```python
from build123d import *

# Parameters (mm, degrees)
SKETCH1_R           = 1.5
SKETCH1_W           = 16
SKETCH1_H           = 16
BOSS_EXTRUDE1_DEPTH = 4
BOSS_EXTRUDE2_START = 2
BOSS_EXTRUDE2_DEPTH = 2


with BuildPart() as part:
    # Sketch1 → Boss-Extrude1 (new body)
    with BuildSketch(Plane(origin=(0, 0, 0), x_dir=(1, 0, 0), z_dir=(0, 1, 0))):
        with BuildLine():
            Line((-2, 18), (18, 18))
            Line((18, 18), (18, -2))
            Line((18, -2), (-2, -2))
            Line((-2, -2), (-2, 4.5))
            Line((-2, 4.5), (-4, 4.5))
            ThreePointArc((-4, 4.5), (-7.5, 8), (-4, 11.5))
            Line((-4, 11.5), (-2, 11.5))
            Line((-2, 11.5), (-2, 18))
        make_face()
        with Locations(Location((-4, 8, 0), (0, 0, 270))):
            Circle(SKETCH1_R, mode=Mode.SUBTRACT)
        with Locations((8, 8)):
            Rectangle(SKETCH1_W, SKETCH1_H, mode=Mode.SUBTRACT)
    extrude(amount=BOSS_EXTRUDE1_DEPTH)

    # Sketch2 → Boss-Extrude2 (add)
    with BuildSketch(Plane.XZ.offset(BOSS_EXTRUDE2_START)):
        with BuildLine():
            Line((18, 2), (18, -18))
            Line((18, -18), (-2, -18))
            Line((-2, -18), (-2, -11.5))
            Line((-2, -11.5), (-4, -11.5))
            ThreePointArc((-4, -11.5), (-7.5, -8), (-4, -4.5))
            Line((-4, -4.5), (-2, -4.5))
            Line((-2, -4.5), (-2, 2))
            Line((-2, 2), (18, 2))
        make_face()
    extrude(amount=-BOSS_EXTRUDE2_DEPTH)


solid = part.part
```
The listing builds one solid part. Answer for the finished solid, in the listing's coordinates (mm). A direction names the side the tool comes from. Give positions to 0.01 mm unless a question says otherwise; leave off trailing zeros. Order: outer loops, then holes, each group sorted by start corner. A loop starts at its lowest first (then second) coordinate and runs counter-clockwise, first axis right, second up. Notation, with made-up numbers: (4.25, 63.5) - (63.25, 63.5) arc R13 ccw to (63.25, 75.5) - close; hole circle Ø4 at (80, 56.25). An arc over 180 degrees is marked (long way). Answer in a Markdown table with one row per item. Add a question column.
Q1. Given P1, Ø1.5, axis at x = -4.5, z = -14.5, coming from the +Y side; P2, Ø0.6, axis at x = -3.5, y = 0, coming from the +Z side; P3, Ø1.5, axis at y = 1.5, z = -11.5, coming from the -X side; P4, Ø1.5, axis at x = 11, z = -1.5, coming from the +Y side, each flat-ended and moving along its own axis, determine where each tip first touches the part or whether it passes through.
Q2. The part is cut by section B-B (x = 11.5). Determine the outline of the cut face in (y, z), then the cut area to 3 significant figures.
Q3. The part is cut by section A-A (y = 3). Determine the outline of the cut face in (x, z).
Q4. Find the intervals of material crossed by line 1 along X through (y, z) = (1.2, -8); line 2 along Z through (x, y) = (6.75, 3.25); line 3 along X through (y, z) = (0.95, -8.5), in increasing order. Write a range as [from, to].
Q5. Which of the six approach directions +Z, -Z, +X, -X, +Y, -Y give full straight-line access (tool end or side, diameter ignored) to faces 4 (the flat face through (-2, 1, -15)), 5 (the flat face through (-3, 1, -4.5)), 6 (the flat face through (8, 0, -8)), 7 (the flat face through (18, 1, -8)), 8 (the flat face through (8, 1, 2))?
Q6. The part is cut by section D-D (z = -8). Determine the outline of the cut face in (x, y).
Q7. The part is cut by section C-C (z = -1.75). Determine the outline of the cut face in (x, y), then the cut area to 3 significant figures.
Q8. For a pull along Z with two mould halves and no side action, classify faces 1 (the flat face through (-3, 1, -11.5)), 2 (the flat face through (-2, 1, -1)), 3 (the flat face through (8, 2, 0)) as released by +Z, released by -Z, zero draft, split by the parting line, or undercut.
Determined:
| question | item | result |
|---|---|---|
| 1 | P1 | passes through |
| 1 | P2 | stops at z = -4.5 |
| 1 | P3 | stops at x = -6.17 |
| 1 | P4 | stops at y = 0 |
| 2 | outline | (-2, -18) - (4, -18) - (4, -16) - (0, -16) - (0, 0) - (4, 0) - (4, 2) - (-2, 2) - close |
| 2 | area | 56.0 mm² |
| 3 | outline | (-4, -11.5) - (-2, -11.5) - (-2, -18) - (18, -18) - (18, 2) - (-2, 2) - (-2, -4.5) - (-4, -4.5) arc R3.5 ccw to start; hole circle Ø3 at (-4, -8); hole (0, -16) - (16, -16) - (16, 0) - (0, 0) - close |
| 4 | line 1 | x = [-7.5, -5.5], [-2.5, 0], [16, 18] |
| 4 | line 2 | z = [-18, -16], [0, 2] |
| 4 | line 3 | x = [-7.46, -5.41], [-2.59, 0], [16, 18] |
| 5 | face 4 | -Z, -X, +Y, -Y |
| 5 | face 5 | +Z, -X, +Y, -Y |
| 5 | face 6 | +Y |
| 5 | face 7 | +Z, -Z, +X, +Y, -Y |
| 5 | face 8 | +Z, +X, -X, +Y, -Y |
| 6 | outline | (-7.5, -2) - (18, -2) - (18, 4) - (16, 4) - (16, 0) - (0, 0) - (0, 4) - (-2.5, 4) - (-2.5, 0) - (-5.5, 0) - (-5.5, 4) - (-7.5, 4) - close |
| 7 | outline | (-2, -2) - (18, -2) - (18, 4) - (16, 4) - (16, 0) - (0, 0) - (0, 4) - (-2, 4) - close |
| 7 | area | 56.0 mm² |
| 8 | face 1 | released by -Z |
| 8 | face 2 | zero draft |
| 8 | face 3 | undercut |
